For this review, take the finished solid that the model builds, in its own axes (mm). A direction names the side the tool comes from. Give positions to 0.01 mm unless a question says otherwise; leave off trailing zeros. Write each loop counter-clockwise with the first axis right and the second up, starting at its lowest first coordinate (ties: lowest second). Pieces come first, ordered by that corner, then holes.
Autodesk Inventor part; units mm, degrees
ref_plane "YZ Plane" through (0, 0, 0) normal (1, 0, 0) x (0, 1, 0)
ref_plane "XZ Plane" through (0, 0, 0) normal (0, 1, 0) x (-1, 0, 0)
ref_plane "XY Plane" through (0, 0, 0) normal (0, 0, 1) x (1, 0, 0)
sketch "Sketch1" plane through (0, 0, 0) normal (1, 0, 0) x (0, 1, 0)
  circle A0 centre (0, 0) radius 3.175
  dimension "d0" = 6.35
extrude "Extrusion1" add sketch "Sketch1" along normal blind 63.5
thread "Thread1"
sketch "Sketch2" plane through (63.5, 0, 0) normal (1, 0, 0) x (0, 0, -1)
  circle A0 centre (0, 0) radius 6.35
  line L0 (6.35, 0) -> (3.175, -5.4993)
  line L1 (3.175, -5.4993) -> (-3.175, -5.4993)
  line L2 (-3.175, -5.4993) -> (-6.35, 0)
  line L3 (-6.35, 0) -> (-3.175, 5.4993)
  line L4 (-3.175, 5.4993) -> (3.175, 5.4993)
  line L5 (3.175, 5.4993) -> (6.35, 0)
  dimension "d5" = 12.7
extrude "Extrusion2" add sketch "Sketch2" along normal blind 3.9688 contours L0 L1 L2 L3 L4 L5
properties part number "support bolt"
(1) We need section B-B (y = 1). Write out the cut boundary in (x, z), and give its area (3 significant figures).
(2) Tool access review of faces 1 (the cylindrical face through (31.31, -0.69, 3.1)), 2 (the flat face through (67.469, 0, 0)): name each direction out of +Z, -Z, +X, -X, +Y, -Y from which nothing blocks a thin tool from reaching the whole face with its end or side.
(3) Clearance check with flat-ended pins moving along their axes: pin 1 Ø3 at (x, y) = (52.5, 1) entering from -Z (3 decimals); pin 2 Ø6 at (x, y) = (27.5, 0) entering from +Z (3 decimals); pin 3 Ø1 at (x, z) = (50, -2.5) entering from -Y. State where each tip first meets the part, or that it passes through.
(4) We need section A-A (z = 0). Write out the cut boundary in (x, y) (3 decimals).
(5) We need section C-C (x = 46). Write out the cut boundary in (y, z) (3 decimals), and give its area (3 significant figures).
(6) For L1, parallel to X at y = -3.25, z = 2.75; L2, parallel to Z at x = 15, y = 0 (3 decimals); L3, parallel to Y at x = 61, z = 0.25, list the stretches that pass through material, from the lowest coordinate up.
(7) We need section D-D (y = -3.75). Write out the cut boundary in (x, z), and give its area (3 significant figures).
The answers:
1. outline: (0, -3.01) - (63.5, -3.01) - (63.5, -5.77) - (67.47, -5.77) - (67.47, 5.77) - (63.5, 5.77) - (63.5, 3.01) - (0, 3.01) - close
1. area: 429 mm2
2. face 1: -X
2. face 2: +Z, -Z, +X, +Y, -Y
3. pin 1: stops at z = -3.175
3. pin 2: stops at z = 3.175
3. pin 3: stops at y = -2.47
4. outline: (0, -3.175) - (63.5, -3.175) - (63.5, -5.499) - (67.469, -5.499) - (67.469, 5.499) - (63.5, 5.499) - (63.5, 3.175) - (0, 3.175) - close
5. outline: circle Ø6.35 at (0, 0)
5. area: 31.7 mm2
6. L1: x = 63.5 to 67.47
6. L2: z = -3.175 to 3.175
6. L3: y = -3.17 to 3.17
7. outline: (63.5, -4.18) - (67.47, -4.18) - (67.47, 4.18) - (63.5, 4.18) - close
7. area: 33.2 mm2
